Geometry: final body of the model. Coordinates: model frame, mm. A direction names the side the tool comes from. Coordinates: 2 decimals unless noted, no trailing zeros. Write each loop counter-clockwise with the first axis right and the second up, starting at its lowest first coordinate (ties: lowest second). Pieces come first, ordered by that corner, then holes. Notation, with made-up numbers: M 58.25,83.5 L 108.25,83.5 A26 cw 108.25,122.5 Z; hole C 33.5,4 d5. An arc over 180 degrees is marked long. Write item = value, one per line. Start each with the question number.
Item 1: Reachability of faces 1 (the flat face through (10, 5, 0.5)), 2 (the flat face through (-6.036, 0, 0.5)), 3 (the flat face through (-7.5, 13.5, 0.5)) from +Z, -Z, +X, -X, +Y, -Y: full face, straight path, thin tool, end or side. Return the list, or none.
Item 2: Section C-C on z = 0.25. Output: boundary loops of the cut face in (x, y).
Item 3: Section B-B on y = 11.75. Output: boundary loops of the cut face in (x, z).
Item 4: Ray query, L1, parallel to Y at x = -13.5, z = 0.25; L2, parallel to Y at x = 10, z = 0.1; L3, parallel to X at y = -4.5, z = 0.1. Return the intervals inside material, ascending. Write a range as [from, to].
Item 5: Section D-D on y = -1. Output: boundary loops of the cut face in (x, z), plus the area to 3 significant figures.
Item 6: Pull-direction query (X, two-part tool) for faces 4 (the cylindrical face through (0, -8.5, 0.5)), 5 (the flat face through (-16.036, 5, 0.5)), 6 (the flat face through (-13.6, 7.5, 0.5)), 7 (the flat face through (-1.268, 8.13, 0.493)); classes: +X half, -X half, draft (parallel to the pull), parting line (faces both ways), or undercut.
Item 7: First-contact query: pin 1 Ø0.5 at (y, z) = (1, 0.5) entering from +X. Flat tip, straight axial feed; report the tip coordinate or a pass-through.
Item 8: Section A-A on x = 9.5. Output: boundary loops of the cut face in (y, z).
from build123d import *

# Parameters (mm, degrees)
PAD_DEPTH = 1


with BuildPart() as part:
    # Sketch → Pad (new body)
    with BuildSketch(Plane.XY):
        with BuildLine():
            Line((-16.035534, -10), (-16.035534, -2.5))
            Line((-16.035534, -2.5), (-6.035534, -2.5))
            Line((-6.035534, -2.5), (-6.035534, 2.5))
            Line((-6.035534, 2.5), (-16.035534, 2.5))
            Line((-16.035534, 2.5), (-16.035534, 7.5))
            Line((-16.035534, 7.5), (-11.035534, 7.5))
            Line((-11.035534, 7.5), (-7.5, 11.035534))
            Line((-7.5, 11.035534), (-7.5, 16.035534))
            Line((-7.5, 16.035534), (-2.5, 16.035534))
            Line((-2.5, 16.035534), (0, 0))
            Line((0, 0), (2.5, 16.035534))
            Line((2.5, 16.035534), (12.5, 16.035534))
            Line((12.5, 16.035534), (12.5, 5))
            Line((12.5, 5), (7.5, 5))
            Line((7.5, 5), (7.5, -5))
            Line((7.5, -5), (12.5, -5))
            Line((12.5, -5), (12.5, -10))
            Line((12.5, -10), (1.5, -10))
            ThreePointArc((1.5, -10), (0, -8.5), (-1.5, -10))
            Line((-1.5, -10), (-16.035534, -10))
        make_face()
    extrude(amount=PAD_DEPTH)


solid = part.part
Responses:
q1.face_1 = +Z, -Z, +X
q1.face_2 = +Z, -Z, -X
q1.face_3 = +Z, -Z, -X, +Y
q2.outline = M -16.04,-10 L -1.5,-10 A1.5 cw 1.5,-10 L 12.5,-10 L 12.5,-5 L 7.5,-5 L 7.5,5 L 12.5,5 L 12.5,16.04 L 2.5,16.04 L 0,0 L -2.5,16.04 L -7.5,16.04 L -7.5,11.04 L -11.04,7.5 L -16.04,7.5 L -16.04,2.5 L -6.04,2.5 L -6.04,-2.5 L -16.04,-2.5 Z
q3.outline = M -7.5,0 L -1.83,0 L -1.83,1 L -7.5,1 Z; M 1.83,0 L 12.5,0 L 12.5,1 L 1.83,1 Z
q4.L1 = [-10, -2.5], [2.5, 7.5]
q4.L2 = [-10, -5], [5, 16.04]
q4.L3 = [-16.04, 7.5]
q5.outline = M -6.04,0 L 7.5,0 L 7.5,1 L -6.04,1 Z
q5.area = 13.5 mm²
q6.face_4 = undercut
q6.face_5 = -X half
q6.face_6 = draft
q6.face_7 = undercut
q7.pin_1 = 7.5
q8.outline = M -10,0 L -5,0 L -5,1 L -10,1 Z; M 5,0 L 16.04,0 L 16.04,1 L 5,1 Z
